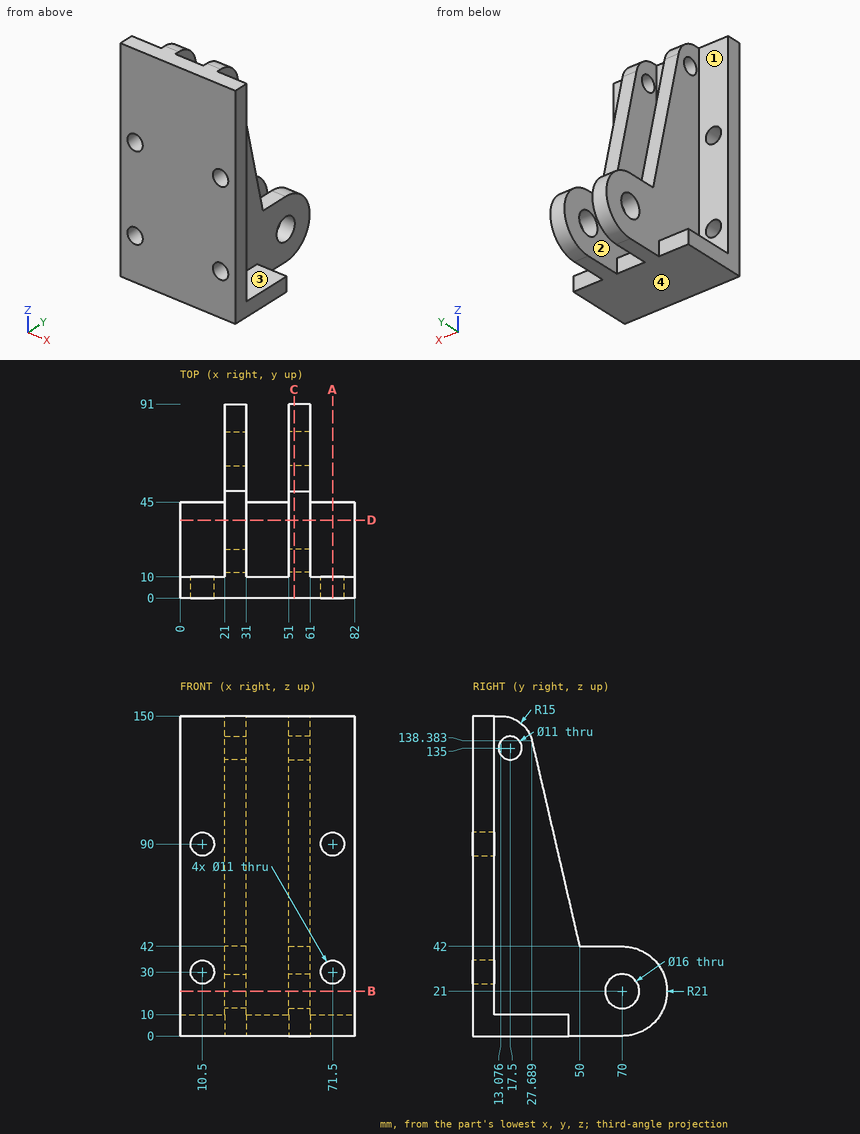
Source: three-view drawing plus pictorial views. Frame: mm from the lowest corner of the part. A direction names the side the tool comes from. Round coordinates to 2 decimals unless told otherwise and drop trailing zeros. Order: outer loops, then holes, each group sorted by start corner. A loop starts at its lowest first (then second) coordinate and runs counter-clockwise, first axis right, second up. Notation, with made-up numbers: M 4.25,85.25 L 30.25,85.25 A33 cw 30.25,120.25 Z; hole C 55,83 d2. An arc over 180 degrees is marked long. One line per item, written item: value.
(1) Line query: probe 1 along X at (y, z) = (3, 30); probe 2 along Z at (x, y) = (10, 4); probe 3 along X at (y, z) = (19, 79.5). Output: solid intervals per line, ascending. Write a range as [from, to].
Result sheet:
probe 1: [0, 5], [16, 66], [77, 82]
probe 2: [0, 24.52], [35.48, 84.52], [95.48, 150]
probe 3: [21, 31], [51, 61]
(2) Cut plane D-D (y = 36.5). Return the cut outline in (x, z), and give its area (3 significant figures).
Result sheet:
outline: M 0,0 L 82,0 L 82,10 L 61,10 L 61,100.32 L 51,100.32 L 51,10 L 31,10 L 31,100.32 L 21,100.32 L 21,10 L 0,10 Z
area: 2,630 mm2
(3) Pin query (flat end, axial travel): P1, Ø8, axis at x = 57.5, y = 63, coming from the +Z side; P2, Ø11, axis at x = 67, z = 4, coming from the +Y side; P3, Ø1, axis at x = 58.5, z = 77, coming from the +Y side; P4, Ø10, axis at x = 43, y = 50.5, coming from the -Z side. Return the tip coordinate at first contact, or that it passes through.
Result sheet:
P1: z = 42
P2: y = 45
P3: y = 42.01
P4: through
(4) Reachability of the marked faces 1, 2, 3 and 4 from +Z, -Z, +X, -X, +Y, -Y: full face, straight path, thin tool, end or side. Return the list, or none.
Result sheet:
face 1: +Z, -X, +Y
face 2: +Z, +Y
face 3: +Z, +X, +Y
face 4: -Z, +X, -X, +Y, -Y
(5) Cut plane A-A (x = 71.5). Return the cut outline in (y, z), and give its area (3 significant figures).
Result sheet:
outline: M 0,0 L 45,0 L 45,10 L 10,10 L 10,24.5 L 0,24.5 Z; M 0,35.5 L 10,35.5 L 10,84.5 L 0,84.5 Z; M 0,95.5 L 10,95.5 L 10,150 L 0,150 Z
area: 1,630 mm2
(6) Cut plane C-C (x = 53.5). Return the cut outline in (y, z) (1 decimal), and give its area (3 significant figures).
Result sheet:
outline: M 0,0 L 70,0 A21 ccw 70,42 L 50,42 L 27.7,138.4 A15 ccw 13.1,150 L 0,150 Z; hole C 17.5,135 d11; hole C 70,21 d16
area: 7,360 mm2
(7) Cut plane B-B (z = 21). Return the cut outline in (x, y).
Result sheet:
outline: M 0,0 L 82,0 L 82,10 L 61,10 L 61,62 L 51,62 L 51,10 L 31,10 L 31,62 L 21,62 L 21,10 L 0,10 Z; M 21,78 L 31,78 L 31,91 L 21,91 Z; M 51,78 L 61,78 L 61,91 L 51,91 Z
